Autodesk Inventor part; units mm, degrees
ref_plane "YZ Plane" through (0, 0, 0) normal (1, 0, 0) x (0, 1, 0)
ref_plane "XZ Plane" through (0, 0, 0) normal (0, 1, 0) x (-1, 0, 0)
ref_plane "XY Plane" through (0, 0, 0) normal (0, 0, 1) x (1, 0, 0)
sketch "Sketch1" plane through (0, 0, 0) normal (0, 0, 1) x (1, 0, 0)
  circle A0 centre (0, 0) radius 31.830989
  circle A1 centre (0, 0) radius 32.205989
  circle A2 centre (0, 0) radius 31.576989
  dimension "d0" = 63.66198
  dimension "d2" = 0.254
  dimension "d3" = 0.375
sketch "Sketch1 outline for Extrusion1" plane through (0, 0, 0) normal (0, 0, 1) x (1, 0, 0)
  circle A0 centre (0, 0) radius 32.205989
  circle A1 centre (0, 0) radius 31.576989
extrude "Extrusion1" add sketch "Sketch1 outline for Extrusion1" along normal blind 6
sketch "Sketch2" plane through (0, 0, 6) normal (0, 0, 1) x (1, 0, 0)
  circle A0 centre (0, 0) radius 32.205989
  line L0 (0, 0) -> (3.816108, 31.979103)
  line L1 (0, 0) -> (3.816108, -31.979103)
  dimension "d6" = 166.39
extrude "Extrusion2" cut sketch "Sketch2" against normal through all contours A0 L1 L0 picked at (21.157827, -2.572713)
sketch "Sketch3" plane through (3.816108, 31.979103, 6) normal (0.9929552, -0.1184906, 0) x (0, 0, -1)
  line L0 (6, 0) -> (6, -0.629)
  line L1 (0, 0) -> (6, 0)
  line L2 (0, -0.629) -> (0, 0)
  line L3 (6, -0.629) -> (0, -0.629)
  point P0 (6, -32.205989)
  point P1 (3, -0.375)
  point P2 (3, -0.629)
  dimension "d9" = 0.254
coil "Coil1" sketch "Sketch3" operation add axis through (3.771674, 31.606745, 3) along (0.9929552, -0.1184906, 0) pitch 371.456 turns 0.25 hand right
sketch "Sketch4" plane through (3.741577, -31.354534, 6) normal (0.9929552, 0.1184906, 0) x (0, 0, -1)
  line L0 (6, 0) -> (6, -0.629)
  line L1 (0, 0) -> (6, 0)
  line L2 (0, -0.629) -> (0, 0)
  line L3 (6, -0.629) -> (0, -0.629)
  point P0 (6, 31.576989)
  point P1 (3, -0.254)
  point P2 (3, 0)
  dimension "d18" = 0.254
coil "Coil2" sketch "Sketch4" operation add axis through (3.771674, -31.606745, 3) along (0.9929552, 0.1184906, 0) pitch 371.456 turns 0.25 hand right
sketch "Sketch5" plane through (95.625991, -17.624366, 3.254) normal (0.9929552, 0.1184906, 0) x (0, 0, -1)
  line L0 (0.629, 0) -> (0.629, -6)
  line L1 (0, 0) -> (0.629, 0)
  line L2 (0, -6) -> (0, 0)
  line L3 (0.629, -6) -> (0, -6)
  line L4 (7.629, 3.824142) -> (7.629, -17.635602)
  point P0 (3.254, 28.830989)
  dimension "d27" = 7
revolve "Revolution1" add sketch "Sketch5" angle 90 about axis through (95.172866, -13.827165, -4.375) along (-0.1184906, 0.9929552, 0)
sketch "Sketch6" plane through (96.336935, 23.582097, 3.375) normal (0.9929552, -0.1184906, 0) x (0, 0, -1)
  line L0 (0.629, 0) -> (0.629, -6)
  line L1 (0, 0) -> (0.629, 0)
  line L2 (0, -6) -> (0, 0)
  line L3 (0.629, -6) -> (0, -6)
  line L4 (-7, 6.068729) -> (-7, -13.038094)
  point P0 (3.375, -34.830989)
  dimension "d29" = 7
revolve "Revolution2" add sketch "Sketch6" angle 90 about axis through (97.056022, 29.608074, 10.375) along (-0.1184906, -0.9929552, 0)
sketch "Sketch9" plane through (96.336935, -23.582097, 2.625) normal (0.1184906, -0.9929552, 0) x (0.9929552, 0.1184906, 0)
  line L0 (7, -7) -> (7.629, -7)
  line L1 (7.629, -7) -> (7.629, -96.263661)
  line L2 (7.629, -96.263661) -> (7, -96.263661)
  line L3 (7, -96.263661) -> (7, -7)
  line L4 (-19.311334, -96.263661) -> (32.837796, -96.263661)
  point P0 (-92.864, -2.625)
extrude "Extrusion5" add sketch "Sketch9" against normal up to surface (6 mm away)
sketch "Sketch8" plane through (96.336935, 23.582097, 3.375) normal (0.1184906, 0.9929552, 0) x (0.9929552, -0.1184906, 0)
  line L0 (7, -7) -> (7.629, -7)
  line L1 (7.629, -7) -> (7.629, -42.986339)
  line L2 (7.629, -42.986339) -> (7, -42.986339)
  line L3 (7, -42.986339) -> (7, -7)
  line L4 (-19.443403, -42.986339) -> (32.667261, -42.986339)
  point P0 (-92.864, 3.375)
extrude "Extrusion4" add sketch "Sketch8" against normal up to surface (6 mm away)
properties part number "end belt"
Can you work these out from the model? Positions are in its coordinate system, mm. A direction names the side the tool comes from. Round coordinates to 2 decimals unless told otherwise and drop trailing zeros. Write each loop counter-clockwise with the first axis right and the second up, starting at its lowest first coordinate (ties: lowest second). Pieces come first, ordered by that corner, then holes. Notation, with made-up numbers: (-15.75, -33) -> (-0.75, -33) arc R23 ccw to (-0.75, 4) -> close; hole circle Ø9 at (-35.5, 64.25). An arc over 180 degrees is marked (long way). Use one line per item in the form item = value. Start each with the question number.
Q1. We'd pull the mould along Y, two halves only. Please class faces 1 (the face through (103.47, 22.73, 22.84)), 2 (the face through (103.47, -22.73, -41.38)), 3 (the face through (-31.57, -0.75, 2.96)), 4 (the face through (-32.197, -0.762, 2.958)): +Y half, -Y half, draft (parallel to the pull), parting line (faces both ways), or undercut.
Q2. If I drill on probe 1 along Y at (x, z) = (0, 3.1); probe 2 along X at (y, z) = (0, 1.5); probe 3 along X at (y, z) = (-10.5, 2), over which ranges is the centre line in solid material (lowest first)? Write a range as [from, to].
Q3. Imagine slicing it at A-A (x = 0). Please give me the cut outline in (y, z), then the cut area to 3 significant figures.
Q4. Imagine slicing it at B-B (y = 0). Please give me the cut outline in (x, z), then the cut area to 3 significant figures.
Q5. Imagine slicing it at C-C (z = -30.5). Please give me the cut outline in (x, y).
Q6. Which directions (+Z, -Z, +X, -X, +Y, -Y) give clear straight access to the entire face, cutting with the end or side of a thin tool? Please do faces 5 (the face through (100.955, 20.052, 5.48)), 6 (the face through (-32, 0, 6)), 7 (the face through (102.937, -19.816, -49.632)), 8 (the face through (102.937, 19.816, 28.62)).
Worked out:
q1.face_1 = +Y half
q1.face_2 = -Y half
q1.face_3 = undercut
q1.face_4 = parting line
q2.probe_1 = [-32.21, -31.58], [31.58, 32.21]
q2.probe_2 = [-32.21, -31.58]
q2.probe_3 = [-30.45, -29.78]
q3.outline = (-32.21, 0) -> (-31.58, 0) -> (-31.58, 6) -> (-32.21, 6) -> close; (31.58, 0) -> (32.21, 0) -> (32.21, 6) -> (31.58, 6) -> close
q3.area = 7.55 mm^2
q4.outline = (-32.21, 0) -> (-31.58, 0) -> (-31.58, 6) -> (-32.21, 6) -> close
q4.area = 3.77 mm^2
q5.outline = (102.58, -16.79) -> (103.29, -22.75) -> (103.91, -22.68) -> (103.2, -16.72) -> close
q6.face_5 = +Z, +Y
q6.face_6 = +Z, -X, +Y, -Y
q6.face_7 = -Z, -X, -Y
q6.face_8 = +Z, -X, +Y
